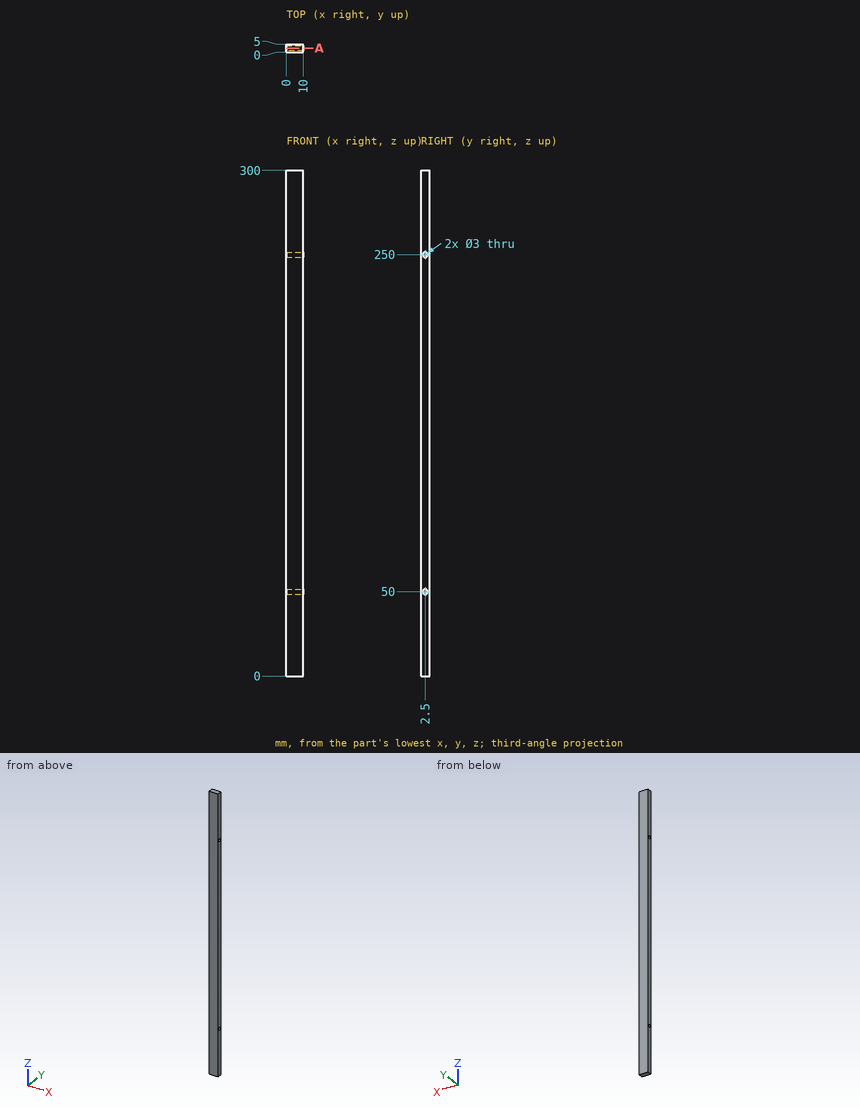
Geometry: see drawing. Coordinates: mm, zero at the bounding-box minimum. Coordinates: 2 decimals unless noted, no trailing zeros. Loops run counter-clockwise (first coordinate to the right, second up) from the corner with the lowest first, then second, coordinate; pieces in that order, holes last. Notation, with made-up numbers: (-19.75, 50) - (-11.75, 50) arc R34 ccw to (-11.75, 88) - close; hole circle Ø10 at (86.5, -12.5). An arc over 180 degrees is marked (long way). Answer as CSV lines item,"result".
1. Section A-A (y = 2.5). Return loops of the section in (x, z), then the cut area to 3 significant figures.
Established:
outline,"(0, 0) - (10, 0) - (10, 48.5) - (0, 48.5) - close; (0, 51.5) - (10, 51.5) - (10, 248.5) - (0, 248.5) - close; (0, 251.5) - (10, 251.5) - (10, 300) - (0, 300) - close"
area,"2,940 mm2"
2. Ray query, line 1 (Z direction, x = 5, y = 2.5); line 2 (Y direction, x = 3, z = 50); line 3 (Z direction, x = 4.5, y = 3.05). Return the intervals inside material, ascending.
Established:
line 1,"z = 0 to 48.5, 51.5 to 248.5, 251.5 to 300"
line 2,"y = 0 to 1, 4 to 5"
line 3,"z = 0 to 48.6, 51.4 to 248.6, 251.4 to 300"
3. Contact query for flat-ended pins moving along their axis: pin 1 (4 mm diameter, centred on x = 1.5, z = 126.5, fed in from -Y); pin 2 (1.8 mm diameter, centred on y = 2.5, z = 250, fed in from -X). Output: stop coordinate, or through.
Established:
pin 1,"stops at y = 0"
pin 2,"passes through"
